from build123d import *

# Parameters (mm, degrees)
SKETCH1_W           = 31.75
SKETCH1_H           = 38.1
BOSS_EXTRUDE1_DEPTH = 6.35
FILLET1_R           = 2.54
SKETCH4_R           = 2.54
CUT_EXTRUDE1_DEPTH  = 6.35


with BuildPart() as part:
    # Sketch1 → Boss-Extrude1 (new body)
    with BuildSketch(Plane.XY):
        with Locations((-25.611666667, 17.674166667)):
            Rectangle(SKETCH1_W, SKETCH1_H)
    extrude(amount=BOSS_EXTRUDE1_DEPTH)

    # Fillet1
    fillet1_edges = [part.edges().sort_by_distance(p)[0] for p in [
        (-9.736666667, 36.724166667, 3.175),
        (-9.736666667, -1.375833333, 3.175),
        (-41.486666667, -1.375833333, 3.175),
        (-41.486666667, 36.724166667, 3.175),
    ]]
    fillet(fillet1_edges, radius=FILLET1_R)

    # Sketch4 → Cut-Extrude1 (cut)
    with BuildSketch(Plane.XY.offset(6.35)):
        with Locations((-14.562666667, 30.374166667)):
            Circle(SKETCH4_R)
        with Locations((-14.562666667, 17.674166667)):
            Circle(SKETCH4_R)
        with Locations((-14.562666667, 4.974166667)):
            Circle(SKETCH4_R)
        with Locations(Location((-36.660666667, 4.974166667, 0), (0, 0, 180))):
            Circle(SKETCH4_R)
        with Locations(Location((-36.660666667, 17.674166667, 0), (0, 0, 180))):
            Circle(SKETCH4_R)
        with Locations(Location((-36.660666667, 30.374166667, 0), (0, 0, 180))):
            Circle(SKETCH4_R)
    extrude(amount=-CUT_EXTRUDE1_DEPTH, mode=Mode.SUBTRACT)


solid = part.part
Verification items for the finished model (mm, model axes). Round coordinates to 2 decimals unless told otherwise and drop trailing zeros. Order: outer loops, then holes, each group sorted by start corner. A loop starts at its lowest first (then second) coordinate and runs counter-clockwise, first axis right, second up.
1. Section check B-B on x = -37. Record the cut outline in (y, z), then the cut area to 3 significant figures.
Final values:
outline: (-1.38, 0) - (2.46, 0) - (2.46, 6.35) - (-1.38, 6.35) - close; (7.49, 0) - (15.16, 0) - (15.16, 6.35) - (7.49, 6.35) - close; (20.19, 0) - (27.86, 0) - (27.86, 6.35) - (20.19, 6.35) - close; (32.89, 0) - (36.72, 0) - (36.72, 6.35) - (32.89, 6.35) - close
area: 146 mm2
2. Release check for a two-part mould opening along X. For faces 1 (the flat face through (-26, 36.724, 3)), 2 (the cylindrical face through (-37.83, 32.63, 3.22)), 3 (the cylindrical face through (-10.5, 36, 3.2)) record: +X half, -X half, draft (parallel to the pull), parting line (faces both ways), or undercut.
Final values:
face 1: draft
face 2: undercut
face 3: +X half
3. Section check A-A on y = 6. Record the cut outline in (x, z), then the cut area to 3 significant figures.
Final values:
outline: (-41.49, 0) - (-38.98, 0) - (-38.98, 6.35) - (-41.49, 6.35) - close; (-34.34, 0) - (-16.89, 0) - (-16.89, 6.35) - (-34.34, 6.35) - close; (-12.24, 0) - (-9.74, 0) - (-9.74, 6.35) - (-12.24, 6.35) - close
area: 143 mm2
4. Section check C-C on z = 3.75. Record the cut outline in (x, y).
Final values:
outline: (-41.49, 1.16) arc R2.54 ccw to (-38.95, -1.38) - (-12.28, -1.38) arc R2.54 ccw to (-9.74, 1.16) - (-9.74, 34.18) arc R2.54 ccw to (-12.28, 36.72) - (-38.95, 36.72) arc R2.54 ccw to (-41.49, 34.18) - close; hole circle Ø5.08 at (-36.66, 4.97); hole circle Ø5.08 at (-36.66, 17.67); hole circle Ø5.08 at (-36.66, 30.37); hole circle Ø5.08 at (-14.56, 4.97); hole circle Ø5.08 at (-14.56, 17.67); hole circle Ø5.08 at (-14.56, 30.37)
5. Section check D-D on x = -13.5. Record the cut outline in (y, z), then the cut area to 3 significant figures.
Final values:
outline: (-1.38, 0) - (2.67, 0) - (2.67, 6.35) - (-1.38, 6.35) - close; (7.28, 0) - (15.37, 0) - (15.37, 6.35) - (7.28, 6.35) - close; (19.98, 0) - (28.07, 0) - (28.07, 6.35) - (19.98, 6.35) - close; (32.68, 0) - (36.72, 0) - (36.72, 6.35) - (32.68, 6.35) - close
area: 154 mm2
6. Thickness scan on L1, parallel to Y at x = -14, z = 4.75; L2, parallel to Y at x = -38, z = 2.25; L3, parallel to X at y = 32, z = 6. Record the ranges inside material, lowest first.
Final values:
L1: y = -1.38 to 2.5, 7.45 to 15.2, 20.15 to 27.9, 32.85 to 36.72
L2: y = -1.38 to 2.82, 7.13 to 15.52, 19.83 to 28.22, 32.53 to 36.72
L3: x = -41.49 to -38.61, -34.71 to -16.51, -12.61 to -9.74
